```python
from build123d import *

# Parameters (mm, degrees)
F0_R     = 0.44
F1_DEPTH = 2.375
F2_W     = 2.5913788058
F2_H     = 0.879
F3_DEPTH = 25
F5_DEPTH = 0.75
F7_DEPTH = 0.75
F8_R     = 0.25
F9_DEPTH = 25
F10_R    = 0.31


with BuildPart() as f1:
    # F0 (on Front) → F1 (new body)
    with BuildSketch(Plane.XZ):
        with BuildLine():
            ThreePointArc((-4.9182944256, 10.6661773273), (-5.0742953332, 10.7208219669), (-5.1620993338, 10.8608675928))
            ThreePointArc((-5.1620993338, 10.8608675928), (-6.7079434791, 11.2153005222), (-6.0202926107, 9.7861773273))
            Line((-6.0202926107, 9.7861773273), (-5.5571346355, 9.7861773273))
            Line((-5.5571346355, 9.7861773273), (1.6257073893, 9.7861773273))
            Line((1.6257073893, 9.7861773273), (1.6257073893, 10.6661773273))
            Line((1.6257073893, 10.6661773273), (-4.9182944256, 10.6661773273))
        make_face()
        with Locations((-6.0202926107, 10.6661773273)):
            Circle(F0_R, mode=Mode.SUBTRACT)
    extrude(amount=F1_DEPTH)

    # F2 (on Top) → F3 (cut)
    with BuildSketch(Plane.XY):
        with Locations((-6.0699820136, -1.1875)):
            Rectangle(F2_W, F2_H)
    extrude(amount=F3_DEPTH, mode=Mode.SUBTRACT)

    # F4 (on face) → F5 (cut)
    with BuildSketch(Plane.XZ.offset(2.375)):
        Polygon((-1.4042926107, 10.6661773273), (-2.6402926107, 10.6661773273), (-2.4042926107, 9.7861773273), (-1.4042926107, 9.7861773273), align=None)
    extrude(amount=-F5_DEPTH, mode=Mode.SUBTRACT)

    # F6 (on face) → F7 (join)
    with BuildSketch(Plane.XZ.offset(2.375)):
        with BuildLine():
            ThreePointArc((-0.8612926107, 12.0361773273), (-1.0020085413, 11.2993410136), (-1.4042926107, 10.6661773273))
            Line((-1.4042926107, 10.6661773273), (-0.1112926107, 10.6661773273))
            Line((-0.1112926107, 10.6661773273), (-0.1112926107, 12.0361773273))
            Line((-0.1112926107, 12.0361773273), (-0.8612926107, 12.0361773273))
        make_face()
    extrude(amount=-F7_DEPTH)

    # F8 (on face) → F9 (cut)
    with BuildSketch(Plane.XY.offset(10.6661773273)):
        with Locations((0.0957073893, -0.88)):
            Circle(F8_R)
    extrude(amount=-F9_DEPTH, mode=Mode.SUBTRACT)

    # F10
    f10_edges = [f1.edges().sort_by_distance(p)[0] for p in [
        (1.625707, -1.1875, 10.666177),
    ]]
    fillet(f10_edges, radius=F10_R)


solid = f1.part
```
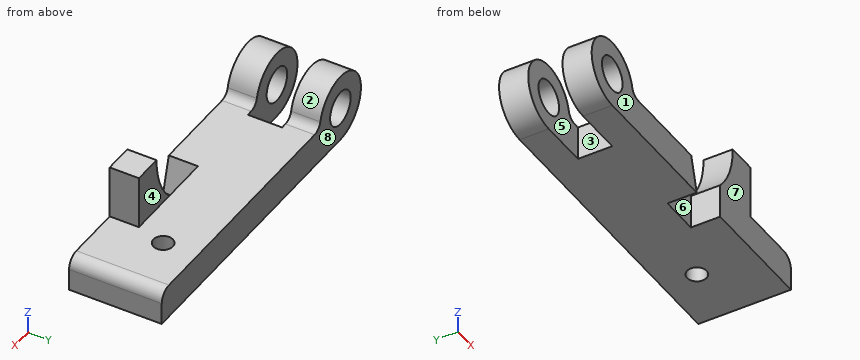
Could you check a few things on this model? Use its own coordinates, in mm. Face numbers are marked on the shaded views. A direction names the side the tool comes from. Coordinates: 2 decimals unless noted, no trailing zeros. Write each loop counter-clockwise with the first axis right and the second up, starting at its lowest first coordinate (ties: lowest second). Pieces come first, ordered by that corner, then holes. Notation, with made-up numbers: (17, 39.25) -> (32, 39.25) arc R10 cw to (32, 53.25) -> close; hole circle Ø11 at (-12.5, 54.25). An arc over 180 degrees is marked (long way). One line per question, with ' | ' between items. Start each with the question number.
1. Will these pins go through, and if not, where does the flat tip stop? P1, Ø1, axis at x = -1, z = 11.5, coming from the +Y side (3 decimals); P2, Ø0.8, axis at y = -2, z = 10, coming from the -X side; P3, Ø1.2, axis at x = -3, y = -1, coming from the +Z side.
2. For the marked faces 4, 5, 6, 7 and 8, which set-ups out of +Z, -Z, +X, -X, +Y, -Y let a thin tool reach every point of the face, with its end or its side?
3. If we section it at C-C (x = -5): Please give me the cut outline in (y, z) (3 decimals), and give its area (3 significant figures).
4. If we section it at D-D (z = 10): Please give me the cut outline in (x, y) (3 decimals), and give its area (3 significant figures).
5. Please list where these lines run through material, in increasing order: line 1 along X through (y, z) = (-2.05, 10.55); line 2 along Z through (x, y) = (-4.5, -1.6); line 3 along Y through (x, z) = (-1.75, 10.05) (3 decimals).
6. If we section it at B-B (y = -0.88): Please give me the cut outline in (x, z).
7. Thinking about a two-plate mould opening in Y: for the marked faces 1, 2 and 3, which applies, pulls with the +Y half, pulls with the -Y half, needs draft (parallel to the pull), parting line crosses it, or undercut?
8. If we section it at A-A (y = -2.05): Please give me the cut outline in (x, z).
Return value:
1) P1: stops at y = -1.625 | P2: stops at x = -6.86 | P3: stops at z = 10.67
2) face 4: +Z, +X, -X, +Y | face 5: +Z, -Z, -X | face 6: +Z, -Y | face 7: +Z, -Z, +X, -X, -Y | face 8: +Z, -Z, +X, -X, +Y
3) outline: (-2.375, 9.786) -> (-1.627, 9.786) -> (-1.627, 10.68) -> (-2.375, 10.68) -> close; (-0.748, 9.786) -> (0, 9.786) -> (0, 10.68) -> (-0.748, 10.68) -> close | area: 1.34 mm²
4) outline: (-6.595, -2.375) -> (-2.462, -2.375) -> (-2.462, -1.625) -> (-1.404, -1.625) -> (-1.404, -2.375) -> (1.626, -2.375) -> (1.626, 0) -> (-6.595, 0) -> (-6.595, -0.748) -> (-4.774, -0.748) -> (-4.774, -1.627) -> (-6.595, -1.627) -> close; hole circle Ø0.5 at (0.096, -0.88) | area: 16.9 mm²
5) line 1: x = -6.89 to -6.44, -5.6 to -2.61, -1.4 to 1.56 | line 2: z = 9.79 to 10.67 | line 3: y = -1.625 to 0
6) outline: (-4.77, 9.79) -> (-0.15, 9.79) -> (-0.15, 10.67) -> (-4.77, 10.67) -> close; (0.35, 9.79) -> (1.63, 9.79) -> (1.63, 10.36) arc R0.31 ccw to (1.32, 10.67) -> (0.35, 10.67) -> close
7) face 1: pulls with the -Y half | face 2: needs draft | face 3: undercut
8) outline: (-6.02, 9.79) -> (-2.4, 9.79) -> (-2.64, 10.67) -> (-4.92, 10.67) arc R0.25 cw to (-5.16, 10.86) arc R0.88 ccw (long way) to start; (-1.4, 9.79) -> (1.63, 9.79) -> (1.63, 10.36) arc R0.31 ccw to (1.32, 10.67) -> (-0.11, 10.67) -> (-0.11, 12.04) -> (-0.86, 12.04) arc R2 cw to (-1.4, 10.67) -> close; hole circle Ø0.88 at (-6.02, 10.67)
